Autodesk Inventor part; units mm, degrees
ref_plane "YZ Plane" through (0, 0, 0) normal (1, 0, 0) x (0, 1, 0)
ref_plane "XZ Plane" through (0, 0, 0) normal (0, 1, 0) x (-1, 0, 0)
ref_plane "XY Plane" through (0, 0, 0) normal (0, 0, 1) x (1, 0, 0)
sketch "Sketch1" plane through (0, 0, 0) normal (0, 0, 1) x (1, 0, 0)
  line L0 (10, -10) -> (-10, -10)
  line L1 (-10, -10) -> (-10, 10)
  line L2 (-10, 10) -> (10, 10)
  line L3 (10, 10) -> (10, -10)
  line L4 (10, -10) -> (-10, 10) construction
  line L5 (-10, -10) -> (10, 10) construction
  line L6 (10, -10) -> (6, -10)
  line L7 (6, -10) -> (6, 10)
  line L8 (6, 10) -> (10, 10)
  line L9 (10, 10) -> (10, -10)
  line L10 (6, 2) -> (4, 2)
  line L11 (4, 2) -> (4, -2)
  line L12 (4, -2) -> (6, -2)
  line L13 (6, -2) -> (6, 2)
  line L14 (0, 10) -> (0, -10)
  point P0 (0, 0)
  dimension "d0" = 20
  dimension "d1" = 20
  dimension "d2" = 4
  dimension "d6" = 2
  dimension "d7" = 2
  dimension "d8" = 4
  dimension "d9" = 2
  dimension "d44" = 6
extrude "Extrusion1" add sketch "Sketch1" along normal blind 5 contours L0 L14 L2 L7 L10 L11 L12
ref_plane "Work Plane1" through (0, 0, 2.5) normal (0, 0, 1) x (1, 0, 0)
sketch "Sketch2" plane through (0, 0, 2.5) normal (0, 0, 1) x (1, 0, 0)
  line L0 (0, 10) -> (0, -10)
  line L1 (0, 2.8868) -> (2.5, 1.4434)
  line L2 (2.5, 1.4434) -> (2.5, -1.4434)
  line L3 (2.5, -1.4434) -> (0, -2.8868)
  line L4 (0, -2.8868) -> (-2.5, -1.4434)
  line L5 (-2.5, -1.4434) -> (-2.5, 1.4434)
  line L6 (-2.5, 1.4434) -> (0, 2.8868)
  point P0 (0, 0)
  point P1 (0, 0)
  dimension "d12" = 5
extrude "Extrusion2" cut sketch "Sketch2" along normal mid plane 1.8
sketch "Sketch3" plane through (0, 0, 5) normal (0, 0, 1) x (1, 0, 0)
  circle A0 centre (0, 0) radius 1.75
  dimension "d15" = 3.5
extrude "Extrusion3" cut sketch "Sketch3" against normal blind 8
sketch "Sketch4" plane through (0, 10, 0) normal (-1, 0, 0) x (0, 0, 1)
  circle A0 centre (2.5, -2.5) radius 0.8
  circle A1 centre (2.5, -17.5) radius 0.8
  line L0 (0, 0) -> (5, 0)
  line L1 (0, 0) -> (0, -8.25)
  line L2 (0, -11.75) -> (0, -20)
  line L3 (0, -20) -> (5, -20)
  point P0 (0, -10)
  dimension "d18" = 1.6
  dimension "d19" = 1.6
  dimension "d20" = 2.5
  dimension "d21" = 2.5
  dimension "d22" = 2.5
  dimension "d23" = 2.5
extrude "Extrusion4" cut sketch "Sketch4" against normal blind 5
thread "Thread1"
thread "Thread2"
sketch "Sketch5" plane through (0, 0, 0) normal (0, 0, -1) x (-1, 0, 0)
  line L0 (-4, -2) -> (-4, 2)
  line L1 (-6, -10) -> (-6, -2)
  line L2 (-4, 2) -> (-6, 2)
  line L3 (-6, 2) -> (-6, -2)
  line L4 (-6, -2) -> (-4, -2)
  line L5 (-4, -2) -> (-4, 2)
  point P0 (0, 0)
extrude "Extrusion5" add sketch "Sketch5" against normal blind 5
sketch "Sketch6" plane through (0, 0, 0) normal (0, 0, -1) x (-1, 0, 0)
  line L0 (-6, -10) -> (-6, 10)
  circle A0 centre (-6, 6) radius 2.5
  line L1 (-6, -9) -> (-3.5, -9)
  line L2 (-3.5, -9) -> (-3.5, -3)
  line L3 (-3.5, -3) -> (-6, -3)
  line L4 (-6, -3) -> (-6, -9)
  line L5 (0, -10) -> (-6, -10)
  line L6 (-6, 10) -> (0, 10)
  point P0 (0, 0)
  point P1 (-6, 8.5)
  point P2 (-6, 3.5)
  dimension "d32" = 2.5
  dimension "d33" = 1
  dimension "d34" = 6
  dimension "d35" = 5
  dimension "d36" = 4
extrude "Extrusion6" cut sketch "Sketch6" against normal blind 5 contours L0 A0 | L0 L3 L2 L1 picked at (-5.3485, 6.5196)
sketch "Sketch7" plane through (6, -3, 0) normal (1, 0, 0) x (0, 0, -1)
  circle A0 centre (-2.5, 3) radius 1.025
  line L0 (-5, 0) -> (-5, 6.5)
  line L1 (0, -7) -> (-5, -7)
  point P0 (0, 3)
  dimension "d39" = 2.5
  dimension "d40" = 10
  dimension "d41" = 2.05
extrude "Extrusion7" cut sketch "Sketch7" against normal blind 12
equation "\"d19\" = d18"
properties part number "POMSliderMotor"
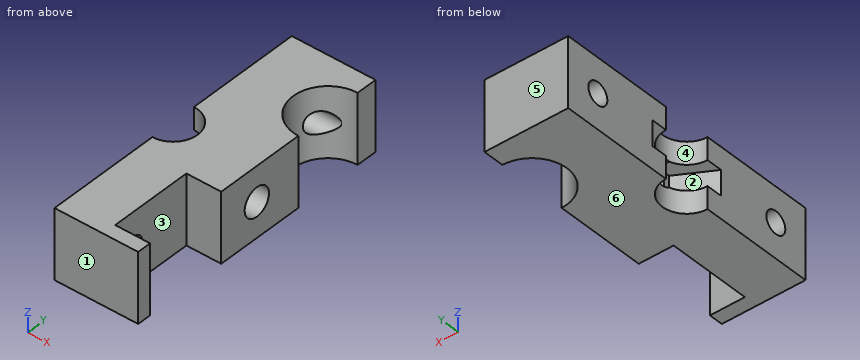
Work out the finished part from the listing and answer in its coordinate system (mm). Face numbers are marked on the shaded views. A direction names the side the tool comes from. Round coordinates to 2 decimals unless told otherwise and drop trailing zeros. Write each loop counter-clockwise with the first axis right and the second up, starting at its lowest first coordinate (ties: lowest second). Pieces come first, ordered by that corner, then holes. Notation, with made-up numbers: (-2.5, 29) - (42.5, 29) arc R16 cw to (42.5, 39) - close; hole circle Ø5 at (4, 57). An arc over 180 degrees is marked (long way). Answer in a Markdown table with one row per item. Add a question column.
1. The mould has two halves that part along Y. Classify the marked faces 4, 5 and 6: +Y half, -Y half, draft (parallel to the pull), parting line (faces both ways), or undercut.
2. A cutting plane is placed at B-B, the plane z = 3.1. Determine the outline of the cut face in (x, y), and give its area (3 significant figures).
3. A cutting plane is placed at C-C, the plane x = 3.75. Determine the outline of the cut face in (y, z) (3 decimals).
4. For the marked faces 1, 2 and 3, determine the directions among +Z, -Z, +X, -X, +Y, -Y from which every point of the face is accessible in a straight line to the end or side of a thin tool.
5. A cutting plane is placed at D-D, the plane x = 1.5. Determine the outline of the cut face in (y, z).
6. Find the intervals of material crossed by line 1 along Z through (x, y) = (2.75, 0) (3 decimals); line 2 along Y through (x, z) = (4.65, 2.5) (3 decimals); line 3 along Y through (x, z) = (4, 0.7), in increasing order. Write a range as from..to.
7. Given pin 1 (1.5 mm diameter, centred on y = -7.5, z = 1.5, fed in from +X); pin 2 (1 mm diameter, centred on y = 7.5, z = 2.5, fed in from +X); pin 3 (1 mm diameter, centred on y = 1, z = 2.5, fed in from -X), each flat-ended and moving along its own axis, determine where each tip first touches the part or whether it passes through.
8. A cutting plane is placed at A-A, the plane y = 7.5. Determine the outline of the cut face in (x, z), and give its area (3 significant figures).
Worked out:
| question | item | result |
|---|---|---|
| 1 | face 4 | undercut |
| 1 | face 5 | +Y half |
| 1 | face 6 | draft |
| 2 | outline | (0, -10) - (6, -10) - (6, -9) - (3.5, -9) - (3.5, -8.03) - (0, -8.03) - close; (0, -6.97) - (3.5, -6.97) - (3.5, -3) - (6, -3) - (6, -0.83) - (2.5, -0.83) - (2.5, -1.44) - (0, -2.89) - close; (0, 2.89) - (2.5, 1.44) - (2.5, 0.83) - (6, 0.83) - (6, 3.5) arc R2.5 cw to (3.7, 6.97) - (0, 6.97) - close; (0, 8.03) - (4.54, 8.03) arc R2.5 cw to (6, 8.5) - (6, 10) - (0, 10) - close |
| 2 | area | 70.6 mm^2 |
| 3 | outline | (-10, 0) - (-9, 0) - (-9, 5) - (-10, 5) - close; (-3, 0) - (4.91, 0) - (4.91, 5) - (-3, 5) - close; (7.09, 0) - (10, 0) - (10, 5) - (7.09, 5) - (7.09, 3.187) arc R0.8 cw (long way) to (7.09, 1.813) - close; hole circle Ø2.05 at (0, 2.5) |
| 4 | face 1 | +Z, -Z, +X, -X, -Y |
| 4 | face 2 | -X |
| 4 | face 3 | +Z, -Z, +X |
| 5 | outline | (-10, 0) - (-0.9, 0) - (-0.9, 1.6) - (-2.02, 1.6) - (-2.02, 3.4) - (-0.9, 3.4) - (-0.9, 5) - (-10, 5) - close; (0.9, 0) - (10, 0) - (10, 5) - (0.9, 5) - (0.9, 3.4) - (2.02, 3.4) - (2.02, 1.6) - (0.9, 1.6) - close; hole circle Ø1.6 at (-7.5, 2.5); hole circle Ø1.6 at (7.5, 2.5) |
| 6 | line 1 | 0..1.475, 3.525..5 |
| 6 | line 2 | -10..-9, -3..-1.025, 1.025..3.896, 8.3..10 |
| 6 | line 3 | -10..-9, -3..4.5, 7.5..10 |
| 7 | pin 1 | x = 3.5 |
| 7 | pin 2 | through |
| 7 | pin 3 | x = 2.4 |
| 8 | outline | (0, 0) - (4, 0) - (4, 1.7) - (0, 1.7) - close; (0, 3.3) - (4, 3.3) - (4, 5) - (0, 5) - close |
| 8 | area | 13.6 mm^2 |
